The listing builds one solid part. Answer for the finished solid, in the listing's coordinates (mm). Face numbers are marked on the shaded views. A direction names the side the tool comes from. Give positions to 0.01 mm unless a question says otherwise; leave off trailing zeros. Write each loop counter-clockwise with the first axis right and the second up, starting at its lowest first coordinate (ties: lowest second). Pieces come first, ordered by that corner, then holes. Notation, with made-up numbers: (65, 24) -> (83, 24) arc R15 cw to (83, 39) -> close; hole circle Ø5 at (84.5, -38). An arc over 180 degrees is marked (long way). Use CSV: the item, a comma, the result in double quotes. Start each with the question number.
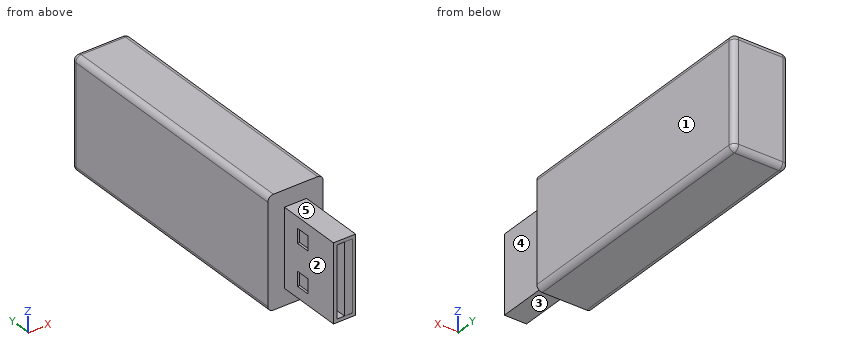
Autodesk Inventor part; units mm, degrees
ref_plane "YZ Plane" through (0, 0, 0) normal (1, 0, 0) x (0, 1, 0)
ref_plane "XZ Plane" through (0, 0, 0) normal (0, 1, 0) x (-1, 0, 0)
ref_plane "XY Plane" through (0, 0, 0) normal (0, 0, 1) x (1, 0, 0)
sketch "Sketch1" plane through (0, 0, 0) normal (0, 1, 0) x (-1, 0, 0)
  line L0 (12.5, 25) -> (-12.5, 25)
  line L1 (-12.5, 25) -> (-12.5, -25)
  line L2 (-12.5, -25) -> (12.5, -25)
  line L3 (12.5, -25) -> (12.5, 25)
  line L4 (17.5, 0) -> (-17.5, 0)
  line L5 (0, -35) -> (0, 35)
  point P0 (0, 0)
  point P1 (12.5, 0)
  point P2 (0, -25)
  dimension "d0" = 50
  dimension "d1" = 25
extrude "Extrusion1" add sketch "Sketch1" along normal mid plane 120
sketch "Sketch2" plane through (0, -60, 0) normal (0, -1, 0) x (1, 0, 0)
  line L0 (-12.5, -25) -> (12.5, -25)
  line L1 (12.5, -25) -> (12.5, 25)
  line L2 (12.5, 25) -> (-12.5, 25)
  line L3 (-12.5, 25) -> (-12.5, -25)
  line L4 (5, 17.5) -> (5, -17.5)
  line L5 (5, -17.5) -> (-5, -17.5)
  line L6 (-5, -17.5) -> (-5, 17.5)
  line L7 (-5, 17.5) -> (5, 17.5)
  point P0 (0, 0)
  dimension "d4" = 10
extrude "Extrusion2" add sketch "Sketch2" along normal blind 30 contours L4 L5 L6 L7
sketch "Sketch3" plane through (0, -90, 0) normal (0, -1, 0) x (1, 0, 0)
  line L0 (5, -17.5) -> (5, 17.5)
  line L1 (5, 17.5) -> (-5, 17.5)
  line L2 (-5, 17.5) -> (-5, -17.5)
  line L3 (-5, -17.5) -> (5, -17.5)
  line L4 (-3.5, -16) -> (0, -16)
  line L5 (0, -16) -> (0, 16)
  line L6 (0, 16) -> (-3.5, 16)
  line L7 (-3.5, 16) -> (-3.5, -16)
  line L8 (-17.5, 0) -> (17.5, 0)
  line L9 (0, -35) -> (0, 35)
  point P0 (0, 0)
  point P1 (-3.5, 0)
  dimension "d7" = 1.5
  dimension "d8" = 1.5
extrude "Extrusion3" cut sketch "Sketch3" against normal blind 30 contours L8 L7 L6 L5 | L5 L4 L7 L8
sketch "Sketch4" plane through (-5, -60, -17.5) normal (-1, 0, 0) x (0, 0, 1)
  line L0 (0, 0) -> (35, 0)
  line L1 (0, 0) -> (0, -30)
  line L2 (35, -30) -> (0, -30)
  line L3 (35, 0) -> (35, -30)
  line L4 (17.5, -60) -> (17.5, 150)
  line L5 (5, -8) -> (11.5, -8)
  line L6 (11.5, -8) -> (11.5, -14.5)
  line L7 (11.5, -14.5) -> (5, -14.5)
  line L8 (5, -14.5) -> (5, -8)
  line L9 (30, -8) -> (23.5, -8)
  line L10 (23.5, -8) -> (23.5, -14.5)
  line L11 (23.5, -14.5) -> (30, -14.5)
  line L12 (30, -14.5) -> (30, -8)
  point P0 (17.5, 60)
  dimension "d11" = 6.5
  dimension "d12" = 6
  dimension "d13" = 8
extrude "Extrusion4" cut sketch "Sketch4" against normal blind 1 contours L5 L6 L7 L8 | L12 L11 L10 L9
fillet "Fillet1" radius 2.5 8 edges at (-12.5, 0, 25) (-12.5, 0, -25) (12.5, 0, 25) (12.5, 0, -25) (0, 60, 25) (-12.5, 60, 0) (0, 60, -25) (12.5, 60, 0)
sketch "Sketch5" plane through (0, -90, 0) normal (0, -1, 0) x (1, 0, 0)
  line L0 (0, -16) -> (-3.5, -16)
  line L1 (-3.5, -16) -> (-3.5, 16)
  line L2 (-3.5, 16) -> (0, 16)
  line L3 (0, 16) -> (0, -16)
  line L4 (5, -17.5) -> (5, 17.5)
  line L5 (5, 17.5) -> (-5, 17.5)
  line L6 (-5, 17.5) -> (-5, -17.5)
  line L7 (-5, -17.5) -> (5, -17.5)
  line L8 (0, -16) -> (3.5, -16)
  line L9 (3.5, -16) -> (3.5, 16)
  line L10 (3.5, 16) -> (0, 16)
  line L11 (0, 16) -> (0, -16)
  point P0 (0, 0)
  dimension "d17" = 1.5
  dimension "d18" = 1.5
extrude "Extrusion5" cut sketch "Sketch5" against normal blind 0.01 contours L3 L10 L9 L8
properties part number "USB_Stick" material "ABS Plastic"
Q1. Straight lines are drawn through the part: L1, parallel to X at y = -76.5, z = 5.5; L2, parallel to Y at x = 0.5, z = 21.5; L3, parallel to Y at x = 1, z = 1. For each, find the intervals that lie inside material, in ascending order.
Q2. For the marked faces 1, 2, 3, 4 and 5, determine the directions among +Z, -Z, +X, -X, +Y, -Y from which every point of the face is accessible in a straight line to the end or side of a thin tool.
Q3. Flat-ended cylindrical pins translate along their axes: pin 1 Ø3.5 at (x, y) = (0, -76.5) entering from -Z; pin 2 Ø1.1 at (x, y) = (-4.5, -72) entering from +Z; pin 3 Ø1 at (y, z) = (-61.5, -17.5) entering from +X. Find the tip coordinate at first contact, or state that the pin passes through.
Q4. Section D-D on z = -20 is taken. Give the vertices of the cut face in (x, y), then the cut area to 3 significant figures.
Q5. Section A-A on y = -78 is taken. Give the vertices of the cut face in (x, z), then the cut area to 3 significant figures.
Output:
1,L1,"-5 to -3.5, 0 to 5"
1,L2,"-60 to 60"
1,L3,"-89.99 to 60"
2,face 1,"+Z, -Z, +X, +Y, -Y"
2,face 2,"+Z, -Z, -X, -Y"
2,face 3,"-Z, +X, -X, -Y"
2,face 4,"+Z, -Z, +X, -Y"
2,face 5,"+Z, +X, -X, -Y"
3,pin 1,"z = -17.5"
3,pin 2,"z = 17.5"
3,pin 3,"x = 5"
4,outline,"(-12.5, -60) -> (12.5, -60) -> (12.5, 57.5) arc R2.5 ccw to (10, 60) -> (-10, 60) arc R2.5 ccw to (-12.5, 57.5) -> close"
4,area,"3,000 mm²"
5,outline,"(-5, -17.5) -> (5, -17.5) -> (5, 17.5) -> (-5, 17.5) -> close; hole (-3.5, -16) -> (0, -16) -> (0, 16) -> (-3.5, 16) -> close"
5,area,"238 mm²"
